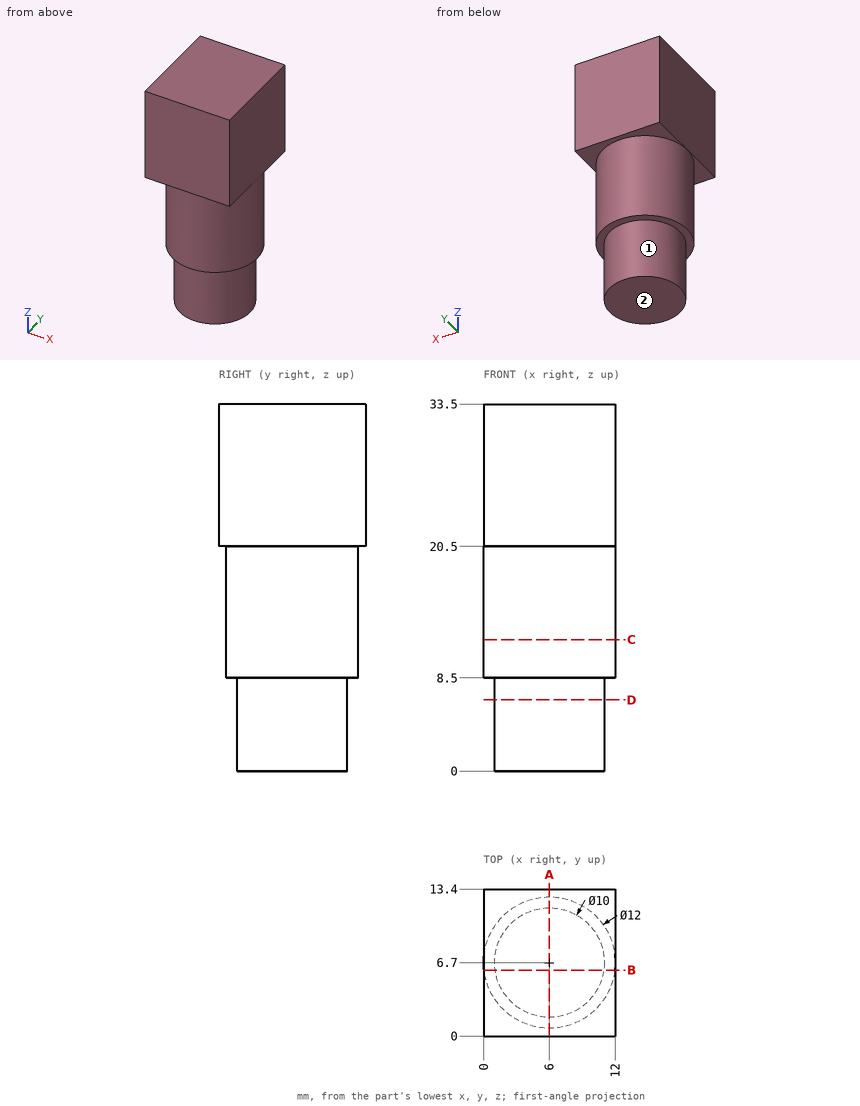
Source: three-view drawing plus pictorial views. Frame: mm from the lowest corner of the part. A direction names the side the tool comes from. Coordinates: 2 decimals unless noted, no trailing zeros. Loops run counter-clockwise (first coordinate to the right, second up) from the corner with the lowest first, then second, coordinate; pieces in that order, holes last. Notation, with made-up numbers: (-8.75, -12.5) - (6.25, -12.5) arc R18 cw to (6.25, 10.5) - close; hole circle Ø2 at (27, -24). An arc over 180 degrees is marked (long way). Answer in a Markdown table with one row per item. Add a question column.
Item 1: Contact query for flat-ended pins moving along their axis: P1, Ø1.5, axis at x = 2, z = 15, coming from the -Y side; P2, Ø5, axis at y = 10.5, z = 16.5, coming from the -X side. Output: stop coordinate, or through.
Item 2: Line query: line 1 along Z through (x, y) = (3.5, 11.5); line 2 along Z through (x, y) = (2.5, 11.75); line 3 along Y through (x, z) = (6.25, 8). Output: solid intervals per line, ascending. Write a range as [from, to].
Item 3: Section query A-A on x = 6. Return the cut outline in (y, z), then the cut area to 3 significant figures.
Item 4: Section query B-B on y = 6. Return the cut outline in (x, z), then the cut area to 3 significant figures.
Item 5: Section query C-C on z = 12. Return the cut outline in (x, y), then the cut area to 3 significant figures.
Item 6: Section query D-D on z = 6.5. Return the cut outline in (x, y).
Item 7: Access query for the marked faces 1 and 2. Directions: +Z, -Z, +X, -X, +Y, -Y. A direction counts if a zero-diameter tool reaches every point of the face in a straight line with its end or side. Return the directions, or none.
Recorded:
| question | item | result |
|---|---|---|
| 1 | P1 | y = 1.66 |
| 1 | P2 | x = 0.14 |
| 2 | line 1 | [8.5, 33.5] |
| 2 | line 2 | [20.5, 33.5] |
| 2 | line 3 | [1.71, 11.69] |
| 3 | outline | (0, 20.5) - (0.7, 20.5) - (0.7, 8.5) - (1.7, 8.5) - (1.7, 0) - (11.7, 0) - (11.7, 8.5) - (12.7, 8.5) - (12.7, 20.5) - (13.4, 20.5) - (13.4, 33.5) - (0, 33.5) - close |
| 3 | area | 403 mm^2 |
| 4 | outline | (0, 20.5) - (0.04, 20.5) - (0.04, 8.5) - (1.05, 8.5) - (1.05, 0) - (10.95, 0) - (10.95, 8.5) - (11.96, 8.5) - (11.96, 20.5) - (12, 20.5) - (12, 33.5) - (0, 33.5) - close |
| 4 | area | 383 mm^2 |
| 5 | outline | circle Ø12 at (6, 6.7) |
| 5 | area | 113 mm^2 |
| 6 | outline | circle Ø10 at (6, 6.7) |
| 7 | face 1 | -Z |
| 7 | face 2 | -Z, +X, -X, +Y, -Y |
